Geometry: final body of the model. Coordinates: model frame, mm. A direction names the side the tool comes from. Give positions to 0.01 mm unless a question says otherwise; leave off trailing zeros. Order: outer loops, then holes, each group sorted by start corner. A loop starts at its lowest first (then second) coordinate and runs counter-clockwise, first axis right, second up. Notation, with made-up numbers: (-14.75, -39.5) - (11.25, -39.5) arc R16 cw to (11.25, -14.5) - close; hole circle Ø6 at (41, 3.5). An arc over 180 degrees is marked (long way). Write item = value, one per line. Start each with the question number.
from build123d import *

# Parameters (mm, degrees)
BOSS_EXTRUDE1_DEPTH = 5
SKETCH4_R           = 2.75
BOSS_EXTRUDE3_DEPTH = 11
SKETCH6_W           = 48
SKETCH6_H           = 10
BOSS_EXTRUDE4_DEPTH = 5
SKETCH7_R           = 3
CUT_EXTRUDE2_DEPTH  = 6
CUT_EXTRUDE3_DEPTH  = 11


with BuildPart() as part:
    # Sketch1 → Boss-Extrude1 (new body, symmetric)
    with BuildSketch(Plane.XY):
        Polygon((-9.5, 17.5), (9.5, 17.5), (9.5, 2.5), (12.5, 2.5), (12.5, -17.5), (-12.5, -17.5), (-12.5, 2.5), (-9.5, 2.5), align=None)
    extrude(amount=BOSS_EXTRUDE1_DEPTH, both=True)

    # Sketch4 → Boss-Extrude3 (add, symmetric)
    with BuildSketch(Plane(origin=(0, 0, 0), x_dir=(0, 0, -1), z_dir=(1, 0, 0))):
        with Locations((0, 12.5)):
            Circle(SKETCH4_R)
    extrude(amount=BOSS_EXTRUDE3_DEPTH, both=True)

    # Sketch6 → Boss-Extrude4 (add)
    with BuildSketch(Plane.XZ.offset(17.5)):
        Rectangle(SKETCH6_W, SKETCH6_H)
    extrude(amount=BOSS_EXTRUDE4_DEPTH)

    # Sketch7 → Cut-Extrude2 (cut, through all)
    with BuildSketch(Plane(origin=(0, -17.5, 0), x_dir=(1, 0, 0), z_dir=(0, 1, 0))):
        with Locations((-18, 0)):
            Circle(SKETCH7_R)
        with Locations((18, 0)):
            Circle(SKETCH7_R)
    extrude(amount=-CUT_EXTRUDE2_DEPTH, mode=Mode.SUBTRACT)

    # Sketch8 → Cut-Extrude3 (cut, through all)
    with BuildSketch(Plane.XY.offset(5)):
        with BuildLine():
            Line((-8, -22.5), (-8, -7.5))
            ThreePointArc((-8, -7.5), (0, 0.5), (8, -7.5))
            Line((8, -7.5), (8, -22.5))
            ThreePointArc((8, -22.5), (0, -30.5), (-8, -22.5))
        make_face()
    extrude(amount=-CUT_EXTRUDE3_DEPTH, mode=Mode.SUBTRACT)


solid = part.part
Q1. Section C-C, the plane x = 18. Return the cut outline in (y, z).
Q2. Set-up query: faces 1 (the cylindrical face through (10.26, 14.359, 2.027)), 2 (the flat face through (11, 13, 0)), 3 (the flat face through (-9.5, 8, 0)), 4 (the flat face through (-12.5, -8, 0)). Return all of +Z, -Z, +X, -X, +Y, -Y with unobstructed straight access to the full face (end or side cutting, diameter ignored); none if empty.
Q3. Section A-A, the plane y = -15.5. Return the cut outline in (x, z).
Q4. Section B-B, the plane z = 0. Count the separate pieces of the cut face and the enclosed holes in it, then the cut area to 3 significant figures.
Q5. Material intervals for line 1 along X through (y, z) = (-19.2, 0); line 2 along Z through (x, y) = (-18, -19); line 3 along X through (y, z) = (-12, -1.5), sorted ascending. Write a range as from..to.
Q6. Pull-direction query (X, two-part tool) for faces 5 (the flat face through (-11, 13, 0)), 6 (the flat face through (-8, -15, 0)), 7 (the flat face through (11, 2.5, 0)); classes: +X half, -X half, draft (parallel to the pull), parting line (faces both ways), or undercut.
Q7. Section D-D, the plane y = 12.5. Return the cut outline in (x, z), then the cut area to 4 significant figures.
Q8. Contact query for flat-ended pins moving along their axis: pin 1 (3 mm diameter, centred on y = -12.5, z = -1, fed in from +X); pin 2 (6 mm diameter, centred on x = -4.5, y = -14.5, fed in from -Z); pin 3 (1.5 mm diameter, centred on x = 11, z = 1, fed in from +Y); pin 4 (6 mm diameter, centred on y = 13.5, z = 1.5, fed in from -X). Output: stop coordinate, or through.
The answers:
q1.outline = (-22.5, -5) - (-17.5, -5) - (-17.5, -3) - (-22.5, -3) - close; (-22.5, 3) - (-17.5, 3) - (-17.5, 5) - (-22.5, 5) - close
q2.face_1 = +X
q2.face_2 = +Z, -Z, +X, +Y
q2.face_3 = -X
q2.face_4 = +Z, -Z, -X, +Y
q3.outline = (-12.5, -5) - (-8, -5) - (-8, 5) - (-12.5, 5) - close; (8, -5) - (12.5, -5) - (12.5, 5) - (8, 5) - close
q4.separate_pieces = 3
q4.enclosed_holes = 0
q4.area = 641 mm²
q5.line_1 = -24..-21, -15..-8, 8..15, 21..24
q5.line_2 = -5..-3, 3..5
q5.line_3 = -12.5..-8, 8..12.5
q6.face_5 = -X half
q6.face_6 = undercut
q6.face_7 = draft
q7.outline = (-11, -2.75) - (-9.5, -2.75) - (-9.5, -5) - (9.5, -5) - (9.5, -2.75) - (11, -2.75) - (11, 2.75) - (9.5, 2.75) - (9.5, 5) - (-9.5, 5) - (-9.5, 2.75) - (-11, 2.75) - close
q7.area = 206.5 mm²
q8.pin_1 = 12.5
q8.pin_2 = through
q8.pin_3 = 15.24
q8.pin_4 = -11
